The model under review builds one solid part; all positions refer to its coordinate system, in mm. Face numbers are marked on the shaded views. Round coordinates to 2 decimals unless told otherwise and drop trailing zeros. Order: outer loops, then holes, each group sorted by start corner. A loop starts at its lowest first (then second) coordinate and runs counter-clockwise, first axis right, second up. Notation, with made-up numbers: M 88,13 L 147,13 A33 ccw 147,49 Z; hole C -18.5,12.25 d8. An arc over 180 degrees is marked long. Use a Markdown table: item, result. Add a question column.
1. The part is to be moulded in two halves that separate along Y. For the marked faces 1, 2 and 3, say which applies: +Y half, -Y half, draft (parallel to the pull), parting line (faces both ways), or undercut.
2. Consider section B-B on z = -0.15. State the section outline as (x, y) points (3 decimals), then the cut area to 3 significant figures.
3. Consider section A-A on y = -21. State the section outline as (x, z) points, then the cut area to 3 significant figures.
4. To check wall thickness, follow probe 1 along Y at (x, z) = (0, 0.65) (3 decimals); probe 2 along Y at (x, z) = (-2.5, -0.2) (3 decimals); probe 3 along X at (y, z) = (-16, -0.15). State the ranges of each line that lie inside material, in increasing order.
5. Consider section D-D on x = -5. State the section outline as (y, z) points.
6. Consider section C-C on x = 0. State the section outline as (y, z) points (3 decimals).
Solid Edge part; units mm, degrees
sketch "Sketch1" plane through (0, 0, 0) normal (0, 0, 1) x (1, 0, 0)
  line L0 (-18.75, -37.5) -> (18.75, -37.5)
  line L1 (18.75, -37.5) -> (18.75, 37.5)
  line L2 (18.75, 37.5) -> (-18.75, 37.5)
  line L3 (-18.75, 37.5) -> (-18.75, -37.5)
  dimension "D1" = 18.75
  dimension "D2" = 18.75
extrude "Protrusion1" add sketch "Sketch1" along normal mid plane 4
sketch "Sketch2" plane through (0, 0, 2) normal (0, 0, 1) x (1, 0, 0)
  line L0 (3.755, -37.5) -> (11.245, -37.5)
  line L1 (11.245, -37.5) -> (11.245, -33.5)
  line L2 (11.245, -33.5) -> (3.755, -33.5)
  line L3 (3.755, -33.5) -> (3.755, -37.5)
  line L4 (-11.245, -37.5) -> (-3.755, -37.5)
  line L5 (-3.755, -37.5) -> (-3.755, -33.5)
  line L6 (-3.755, -33.5) -> (-11.245, -33.5)
  line L7 (-11.245, -33.5) -> (-11.245, -37.5)
  dimension "D1" = 3.755
  dimension "D2" = 11.245
  dimension "D3" = 11.245
  dimension "D4" = 3.755
extrude "Extrusionsausschnitt_1" cut sketch "Sketch2" against normal blind 8
sketch "Sketch3" plane through (0, 0, 2) normal (0, 0, 1) x (1, 0, 0)
  line L0 (-4.125, 18.125) -> (4.125, 18.125)
  line L1 (4.125, 18.125) -> (4.125, 9.875)
  line L2 (4.125, 9.875) -> (-4.125, 9.875)
  line L3 (-4.125, 9.875) -> (-4.125, 18.125)
  dimension "D1" = 4.125
  dimension "D2" = 4.125
extrude "Extrusionsausschnitt_2" cut sketch "Sketch3" against normal blind 44
fillet "Verrundung_1" radius 10 2 edges at (18.75, 37.5, 0) (-18.75, 37.5, 0)
sketch "Sketch4" plane through (0, 0, 2) normal (0, 0, 1) x (1, 0, 0)
  circle A0 centre (0, -21) radius 9
extrude "Extrusionsausschnitt_3" cut sketch "Sketch4" against normal blind 148
properties material "Holz, Kiefer"
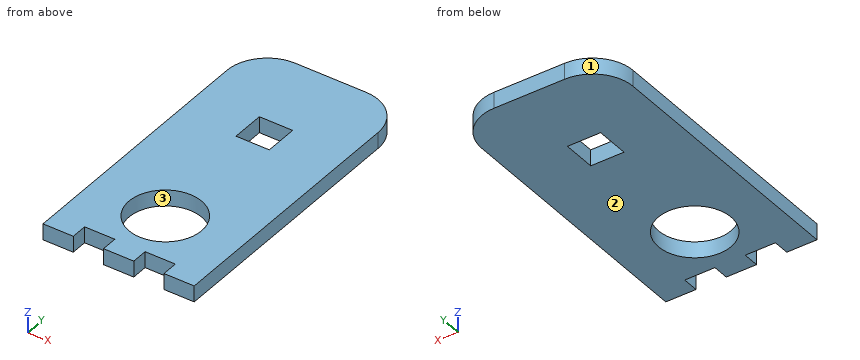
Answer block:
| question | item | result |
|---|---|---|
| 1 | face 1 | +Y half |
| 1 | face 2 | draft |
| 1 | face 3 | undercut |
| 2 | outline | M -18.75,-37.5 L -11.245,-37.5 L -11.245,-33.5 L -3.755,-33.5 L -3.755,-37.5 L 3.755,-37.5 L 3.755,-33.5 L 11.245,-33.5 L 11.245,-37.5 L 18.75,-37.5 L 18.75,27.5 A10 ccw 8.75,37.5 L -8.75,37.5 A10 ccw -18.75,27.5 Z; hole C 0,-21 d18; hole M -4.125,9.875 L 4.125,9.875 L 4.125,18.125 L -4.125,18.125 Z |
| 2 | area | 2,390 mm^2 |
| 3 | outline | M -18.75,-2 L -9,-2 L -9,2 L -18.75,2 Z; M 9,-2 L 18.75,-2 L 18.75,2 L 9,2 Z |
| 3 | area | 78.0 mm^2 |
| 4 | probe 1 | -37.5 to -30, -12 to 9.875, 18.125 to 37.5 |
| 4 | probe 2 | -37.5 to -29.646, -12.354 to 9.875, 18.125 to 37.5 |
| 4 | probe 3 | -18.75 to -7.48, 7.48 to 18.75 |
| 5 | outline | M -33.5,-2 L -28.48,-2 L -28.48,2 L -33.5,2 Z; M -13.52,-2 L 37.5,-2 L 37.5,2 L -13.52,2 Z |
| 6 | outline | M -37.5,-2 L -30,-2 L -30,2 L -37.5,2 Z; M -12,-2 L 9.875,-2 L 9.875,2 L -12,2 Z; M 18.125,-2 L 37.5,-2 L 37.5,2 L 18.125,2 Z |
